Read the model definition and answer for the solid it produces. Units are mm, in the model's axes. A direction names the side the tool comes from. Give positions to 0.01 mm unless a question says otherwise; leave off trailing zeros. Order: outer loops, then holes, each group sorted by start corner. A loop starts at its lowest first (then second) coordinate and runs counter-clockwise, first axis right, second up.
```python
from build123d import *

# Parameters (mm, degrees)
BOSS_EXTRUDE1_DEPTH = 3
SKETCH2_R           = 8
CUT_EXTRUDE2_DEPTH  = 5
SKETCH3_R           = 2
CUT_EXTRUDE3_DEPTH  = 5
SKETCH4_R           = 2
CUT_EXTRUDE4_DEPTH  = 5
SKETCH5_R           = 2
SKETCH5_W           = 4
SKETCH5_H           = 14.81305052
CUT_EXTRUDE5_DEPTH  = 5


with BuildPart() as part:
    # Sketch1 → Boss-Extrude1 (new body)
    with BuildSketch(Plane.XY):
        with BuildLine():
            Line((82, 15), (74.70882917, 15))
            Line((74.70882917, 15), (74.70882917, 39.302424721))
            ThreePointArc((74.70882917, 39.302424721), (73.092812163, 44.753005348), (68.767063336, 48.441939777))
            ThreePointArc((68.767063336, 48.441939777), (55.730177295, 57.736884279), (47.382982574, 71.4))
            ThreePointArc((47.382982574, 71.4), (43.723290865, 76.185352772), (37.978728218, 78))
            Line((37.978728218, 78), (30, 78))
            Line((30, 78), (30, 82))
            ThreePointArc((30, 82), (29.121320344, 84.121320344), (27, 85))
            Line((27, 85), (-27, 85))
            ThreePointArc((-27, 85), (-29.121320344, 84.121320344), (-30, 82))
            Line((-30, 82), (-30, 78))
            Line((-30, 78), (-37.978728218, 78))
            ThreePointArc((-37.978728218, 78), (-43.723290865, 76.185352772), (-47.382982574, 71.4))
            ThreePointArc((-47.382982574, 71.4), (-55.730177295, 57.736884279), (-68.767063336, 48.441939777))
            ThreePointArc((-68.767063336, 48.441939777), (-73.092812163, 44.753005348), (-74.70882917, 39.302424721))
            Line((-74.70882917, 39.302424721), (-74.70882917, 15))
            Line((-74.70882917, 15), (-82, 15))
            ThreePointArc((-82, 15), (-84.121320344, 14.121320344), (-85, 12))
            Line((-85, 12), (-85, -12))
            ThreePointArc((-85, -12), (-84.121320344, -14.121320344), (-82, -15))
            Line((-82, -15), (-74.70882917, -15))
            Line((-74.70882917, -15), (-74.70882917, -39.302424721))
            ThreePointArc((-74.70882917, -39.302424721), (-73.092812163, -44.753005348), (-68.767063336, -48.441939777))
            ThreePointArc((-68.767063336, -48.441939777), (-55.730177295, -57.736884279), (-47.382982574, -71.4))
            ThreePointArc((-47.382982574, -71.4), (-43.723290865, -76.185352772), (-37.978728218, -78))
            Line((-37.978728218, -78), (-30, -78))
            Line((-30, -78), (-30, -82))
            ThreePointArc((-30, -82), (-29.121320344, -84.121320344), (-27, -85))
            Line((-27, -85), (27, -85))
            ThreePointArc((27, -85), (29.121320344, -84.121320344), (30, -82))
            Line((30, -82), (30, -78))
            Line((30, -78), (37.978728218, -78))
            ThreePointArc((37.978728218, -78), (43.723290865, -76.185352772), (47.382982574, -71.4))
            ThreePointArc((47.382982574, -71.4), (55.730177295, -57.736884279), (68.767063336, -48.441939777))
            ThreePointArc((68.767063336, -48.441939777), (73.092812163, -44.753005348), (74.70882917, -39.302424721))
            Line((74.70882917, -39.302424721), (74.70882917, -15))
            Line((74.70882917, -15), (82, -15))
            ThreePointArc((82, -15), (84.121320344, -14.121320344), (85, -12))
            Line((85, -12), (85, 12))
            ThreePointArc((85, 12), (84.121320344, 14.121320344), (82, 15))
        make_face()
    extrude(amount=-BOSS_EXTRUDE1_DEPTH)

    # Sketch2 → Cut-Extrude2 (cut)
    with BuildSketch(Plane.XY):
        Circle(SKETCH2_R)
    extrude(amount=-CUT_EXTRUDE2_DEPTH, mode=Mode.SUBTRACT)

    # Sketch3 → Cut-Extrude3 (cut)
    with BuildSketch(Plane.XY):
        with Locations((81.5, 0)):
            Circle(SKETCH3_R)
        with Locations(Location((-81.5, 0, 0), (0, 0, 180))):
            Circle(SKETCH3_R)
    extrude(amount=-CUT_EXTRUDE3_DEPTH, mode=Mode.SUBTRACT)

    # Sketch4 → Cut-Extrude4 (cut)
    with BuildSketch(Plane.XY):
        with Locations((23, 81.5)):
            Circle(SKETCH4_R)
        with Locations((15, 81.5)):
            Circle(SKETCH4_R)
        with Locations(Location((-15, 81.5, 0), (0, 0, 180))):
            Circle(SKETCH4_R)
        with Locations(Location((-23, 81.5, 0), (0, 0, 180))):
            Circle(SKETCH4_R)
        with Locations((-23, -81.5)):
            Circle(SKETCH4_R)
        with Locations((-15, -81.5)):
            Circle(SKETCH4_R)
        with Locations(Location((15, -81.5, 0), (0, 0, 180))):
            Circle(SKETCH4_R)
        with Locations(Location((23, -81.5, 0), (0, 0, 180))):
            Circle(SKETCH4_R)
    extrude(amount=-CUT_EXTRUDE4_DEPTH, mode=Mode.SUBTRACT)

    # Sketch5 → Cut-Extrude5 (cut)
    with BuildSketch(Plane.XY):
        with Locations((39.243, 41.859)):
            Circle(SKETCH5_R)
        with Locations((39.243, -41.859)):
            Circle(SKETCH5_R)
        with Locations((-39.243, -41.859)):
            Circle(SKETCH5_R)
        with Locations((-39.243, 41.859)):
            Circle(SKETCH5_R)
        with BuildLine():
            Line((-15, -59), (-15, -51))
            ThreePointArc((-15, -51), (-13.828427125, -48.171572875), (-11, -47))
            Line((-11, -47), (11, -47))
            ThreePointArc((11, -47), (13.828427125, -48.171572875), (15, -51))
            Line((15, -51), (15, -59))
            ThreePointArc((15, -59), (13.828427125, -61.828427125), (11, -63))
            Line((11, -63), (-11, -63))
            ThreePointArc((-11, -63), (-13.828427125, -61.828427125), (-15, -59))
        make_face()
        with BuildLine():
            Line((51, 15), (59, 15))
            ThreePointArc((59, 15), (61.828427125, 13.828427125), (63, 11))
            Line((63, 11), (63, -11))
            ThreePointArc((63, -11), (61.828427125, -13.828427125), (59, -15))
            Line((59, -15), (51, -15))
            ThreePointArc((51, -15), (48.171572875, -13.828427125), (47, -11))
            Line((47, -11), (47, 11))
            ThreePointArc((47, 11), (48.171572875, 13.828427125), (51, 15))
        make_face()
        with BuildLine():
            Line((-63, 11), (-63, -11))
            ThreePointArc((-63, -11), (-61.828427125, -13.828427125), (-59, -15))
            Line((-59, -15), (-51, -15))
            ThreePointArc((-51, -15), (-48.171572875, -13.828427125), (-47, -11))
            Line((-47, -11), (-47, 11))
            ThreePointArc((-47, 11), (-48.171572875, 13.828427125), (-51, 15))
            Line((-51, 15), (-59, 15))
            ThreePointArc((-59, 15), (-61.828427125, 13.828427125), (-63, 11))
        make_face()
        with BuildLine():
            Line((-11, 63), (11, 63))
            ThreePointArc((11, 63), (13.828427125, 61.828427125), (15, 59))
            Line((15, 59), (15, 51))
            ThreePointArc((15, 51), (13.828427125, 48.171572875), (11, 47))
            Line((11, 47), (-11, 47))
            ThreePointArc((-11, 47), (-13.828427125, 48.171572875), (-15, 51))
            Line((-15, 51), (-15, 59))
            ThreePointArc((-15, 59), (-13.828427125, 61.828427125), (-11, 63))
        make_face()
        with BuildLine():
            Line((-26.967278586, -57), (-38.5, -57))
            ThreePointArc((-38.5, -57), (-39.560660172, -56.560660172), (-40, -55.5))
            Line((-40, -55.5), (-40, -54.5))
            ThreePointArc((-40, -54.5), (-39.560660172, -53.439339828), (-38.5, -53))
            Line((-38.5, -53), (-26.967278586, -53))
            ThreePointArc((-26.967278586, -53), (-25.906618414, -53.439339828), (-25.467278586, -54.5))
            Line((-25.467278586, -54.5), (-25.467278586, -55.5))
            ThreePointArc((-25.467278586, -55.5), (-25.906618414, -56.560660172), (-26.967278586, -57))
        make_face()
        with Locations((55, 32.59347474)):
            Rectangle(SKETCH5_W, SKETCH5_H)
        with Locations((-55, 32.59347474)):
            Rectangle(SKETCH5_W, SKETCH5_H)
        with BuildLine():
            Line((55.5, -25.18694948), (54.5, -25.18694948))
            ThreePointArc((54.5, -25.18694948), (53.439339828, -25.626289308), (53, -26.68694948))
            Line((53, -26.68694948), (53, -38.5))
            ThreePointArc((53, -38.5), (53.439339828, -39.560660172), (54.5, -40))
            Line((54.5, -40), (55.5, -40))
            ThreePointArc((55.5, -40), (56.560660172, -39.560660172), (57, -38.5))
            Line((57, -38.5), (57, -26.68694948))
            ThreePointArc((57, -26.68694948), (56.560660172, -25.626289308), (55.5, -25.18694948))
        make_face()
        with BuildLine():
            Line((-55.5, -40), (-54.5, -40))
            ThreePointArc((-54.5, -40), (-53.439339828, -39.560660172), (-53, -38.5))
            Line((-53, -38.5), (-53, -26.68694948))
            ThreePointArc((-53, -26.68694948), (-53.439339828, -25.626289308), (-54.5, -25.18694948))
            Line((-54.5, -25.18694948), (-55.5, -25.18694948))
            ThreePointArc((-55.5, -25.18694948), (-56.560660172, -25.626289308), (-57, -26.68694948))
            Line((-57, -26.68694948), (-57, -38.5))
            ThreePointArc((-57, -38.5), (-56.560660172, -39.560660172), (-55.5, -40))
        make_face()
        with BuildLine():
            Line((-25.467278586, 55.5), (-25.467278586, 54.5))
            ThreePointArc((-25.467278586, 54.5), (-25.906618414, 53.439339828), (-26.967278586, 53))
            Line((-26.967278586, 53), (-38.5, 53))
            ThreePointArc((-38.5, 53), (-39.560660172, 53.439339828), (-40, 54.5))
            Line((-40, 54.5), (-40, 55.5))
            ThreePointArc((-40, 55.5), (-39.560660172, 56.560660172), (-38.5, 57))
            Line((-38.5, 57), (-26.967278586, 57))
            ThreePointArc((-26.967278586, 57), (-25.906618414, 56.560660172), (-25.467278586, 55.5))
        make_face()
        with BuildLine():
            Line((26.967278586, 57), (38.5, 57))
            ThreePointArc((38.5, 57), (39.560660172, 56.560660172), (40, 55.5))
            Line((40, 55.5), (40, 54.5))
            ThreePointArc((40, 54.5), (39.560660172, 53.439339828), (38.5, 53))
            Line((38.5, 53), (26.967278586, 53))
            ThreePointArc((26.967278586, 53), (25.906618414, 53.439339828), (25.467278586, 54.5))
            Line((25.467278586, 54.5), (25.467278586, 55.5))
            ThreePointArc((25.467278586, 55.5), (25.906618414, 56.560660172), (26.967278586, 57))
        make_face()
        with BuildLine():
            Line((40, -55.5), (40, -54.5))
            ThreePointArc((40, -54.5), (39.560660172, -53.439339828), (38.5, -53))
            Line((38.5, -53), (26.967278586, -53))
            ThreePointArc((26.967278586, -53), (25.906618414, -53.439339828), (25.467278586, -54.5))
            Line((25.467278586, -54.5), (25.467278586, -55.5))
            ThreePointArc((25.467278586, -55.5), (25.906618414, -56.560660172), (26.967278586, -57))
            Line((26.967278586, -57), (38.5, -57))
            ThreePointArc((38.5, -57), (39.560660172, -56.560660172), (40, -55.5))
        make_face()
    extrude(amount=-CUT_EXTRUDE5_DEPTH, mode=Mode.SUBTRACT)


solid = part.part
```
1) A tool of negligible diameter and unlimited length cuts with its end or side. For faces 4 (the face through (48.203, -13.859, -1.479)), 5 (the face through (55.58, -57.9, -1.48)), from which of +Z, -Z, +X, -X, +Y, -Y can it reach the whole face along a straight path? Write none if from no direction.
Final values:
face 4: +Z, -Z
face 5: +Z, -Z, +X, -Y
2) Given pin 1 (3.5 mm diameter, centred on x = 15, y = -81.5, fed in from +Z); pin 2 (0.9 mm diameter, centred on y = -32, z = -1.5, fed in from +X); pin 3 (1.5 mm diameter, centred on x = -42, z = -2, fed in from +Y); pin 4 (1.5 mm diameter, centred on x = -55, z = -1.5, fed in from -Y), each flat-ended and moving along its own axis, determine where each tip first touches the part or whether it passes through.
Final values:
pin 1: passes through
pin 2: stops at x = 74.71
pin 3: stops at y = 77.45
pin 4: stops at y = -59.42
3) The part is cut by section C-C on y = 0. Determine the outline of the cut face in (x, z), and give its area (3 significant figures).
Final values:
outline: (-85, -3) - (-83.5, -3) - (-83.5, 0) - (-85, 0) - close; (-79.5, -3) - (-63, -3) - (-63, 0) - (-79.5, 0) - close; (-47, -3) - (-8, -3) - (-8, 0) - (-47, 0) - close; (8, -3) - (47, -3) - (47, 0) - (8, 0) - close; (63, -3) - (79.5, -3) - (79.5, 0) - (63, 0) - close; (83.5, -3) - (85, -3) - (85, 0) - (83.5, 0) - close
area: 342 mm2
4) The part is cut by section B-B on x = -23. Determine the outline of the cut face in (y, z).
Final values:
outline: (-85, -3) - (-83.5, -3) - (-83.5, 0) - (-85, 0) - close; (-79.5, -3) - (79.5, -3) - (79.5, 0) - (-79.5, 0) - close; (83.5, -3) - (85, -3) - (85, 0) - (83.5, 0) - close
5) The part is cut by section A-A on y = -30.5. Determine the outline of the cut face in (x, z), and give its area (3 significant figures).
Final values:
outline: (-74.71, -3) - (-57, -3) - (-57, 0) - (-74.71, 0) - close; (-53, -3) - (53, -3) - (53, 0) - (-53, 0) - close; (57, -3) - (74.71, -3) - (74.71, 0) - (57, 0) - close
area: 424 mm2
6) For a pull along X with two mould halves and no side action, classify faces 1 (the face through (43.79, 76.14, -1.48)), 2 (the face through (-23.26, -79.517, -1.479)), 3 (the face through (-43.7, 76.2, -1.5)) as released by +X, released by -X, zero draft, split by the parting line, or undercut.
Final values:
face 1: released by +X
face 2: undercut
face 3: released by -X
7) Consider L1, parallel to Y at x = 23, z = -1; L2, parallel to Y at x = 35.5, z = -2.15; L3, parallel to Y at x = -5, z = -1.95 (3 decimals). Determine where each line is inside the solid, lowest interval first.
Final values:
L1: y = -85 to -83.5, -79.5 to 79.5, 83.5 to 85
L2: y = -78 to -57, -53 to 53, 57 to 78
L3: y = -85 to -63, -47 to -6.245, 6.245 to 47, 63 to 85
8) The part is cut by section D-D on x = 0. Determine the outline of the cut face in (y, z), and give its area (3 significant figures).
Final values:
outline: (-85, -3) - (-63, -3) - (-63, 0) - (-85, 0) - close; (-47, -3) - (-8, -3) - (-8, 0) - (-47, 0) - close; (8, -3) - (47, -3) - (47, 0) - (8, 0) - close; (63, -3) - (85, -3) - (85, 0) - (63, 0) - close
area: 366 mm2
